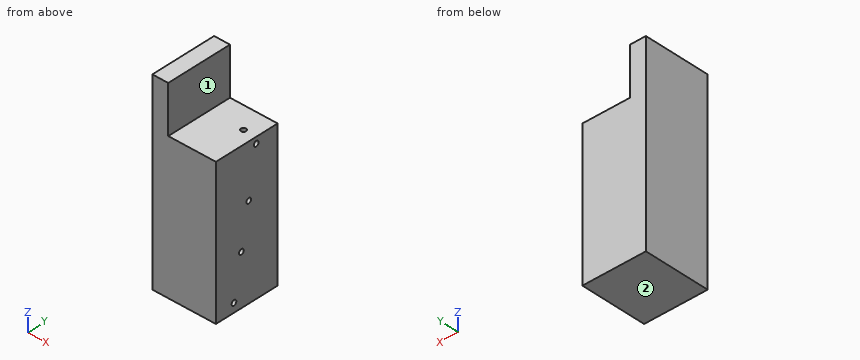
from build123d import *

# Parameters (mm, degrees)
F1_DEPTH = 26.05
F2_R     = 1
F3_DEPTH = 5
F4_R     = 1
F5_DEPTH = 5


with BuildPart() as f1:
    # F0 (on Front) → F1 (new body)
    with BuildSketch(Plane.XZ):
        Polygon((0, 76), (0, 0), (25, 0), (25, 57.25), (6.25, 57.25), (6.25, 76), align=None)
    extrude(amount=-F1_DEPTH)

    # F2 (on face) → F3 (cut)
    with BuildSketch(Plane.YZ.offset(25)):
        with Locations((17, 54.8)):
            Circle(F2_R)
        with Locations((13.875, 36.3)):
            Circle(F2_R)
        with Locations((10.75, 19.9)):
            Circle(F2_R)
        with Locations((7.625, 3.5)):
            Circle(F2_R)
    extrude(amount=-F3_DEPTH, mode=Mode.SUBTRACT)

    # F4 (on face) → F5 (cut)
    with BuildSketch(Plane.XY.offset(57.25)):
        with Locations((20, 17)):
            Circle(F4_R)
    extrude(amount=-F5_DEPTH, mode=Mode.SUBTRACT)


solid = f1.part
Input: part model. Units: mm. Frame: model coordinates. Face numbers are marked on the shaded views. A direction names the side the tool comes from. Coordinates: 2 decimals unless noted, no trailing zeros. Loops run counter-clockwise (first coordinate to the right, second up) from the corner with the lowest first, then second, coordinate; pieces in that order, holes last.
(1) Set-up query: the marked faces 1 and 2. Return all of +Z, -Z, +X, -X, +Y, -Y with unobstructed straight access to the full face (end or side cutting, diameter ignored); none if empty.
(2) First-contact query: pin 1 Ø4 at (x, y) = (8.5, 9) entering from -Z; pin 2 Ø9.5 at (x, y) = (14.5, 8.5) entering from +Z; pin 3 Ø5 at (y, z) = (3.5, 63.5) entering from +X. Flat tips, straight axial feed; report the tip coordinate or a pass-through.
(3) Section A-A on y = 17. Return the cut outline in (x, z).
(4) Section C-C on y = 10.75. Return the cut outline in (x, z).
(5) Section D-D on z = 54.8. Return the cut outline in (x, y), then the cut area to 3 significant figures.
(6) Material intervals for probe 1 along Z at (x, y) = (21.05, 10.75); probe 2 along X at (y, z) = (7, 67); probe 3 along Z at (x, y) = (13, 5.25), sorted ascending.
(7) Section B-B on z = 19.9. Return the cut outline in (x, y).
Data:
1. face 1: +Z, +X, +Y, -Y
1. face 2: -Z, +X, -X, +Y, -Y
2. pin 1: stops at z = 0
2. pin 2: stops at z = 57.25
2. pin 3: stops at x = 6.25
3. outline: (0, 0) - (25, 0) - (25, 53.8) - (21, 53.8) - (21, 52.25) - (19, 52.25) - (19, 57.25) - (6.25, 57.25) - (6.25, 76) - (0, 76) - close; (21, 55.8) - (25, 55.8) - (25, 57.25) - (21, 57.25) - close
4. outline: (0, 0) - (25, 0) - (25, 18.9) - (20, 18.9) - (20, 20.9) - (25, 20.9) - (25, 57.25) - (6.25, 57.25) - (6.25, 76) - (0, 76) - close
5. outline: (0, 0) - (25, 0) - (25, 16) - (20, 16) arc R1 cw to (20, 18) - (25, 18) - (25, 26.05) - (0, 26.05) - close
5. area: 640 mm2
6. probe 1: z = 0 to 18.9, 20.9 to 57.25
6. probe 2: x = 0 to 6.25
6. probe 3: z = 0 to 57.25
7. outline: (0, 0) - (25, 0) - (25, 9.75) - (20, 9.75) - (20, 11.75) - (25, 11.75) - (25, 26.05) - (0, 26.05) - close
